Verification items for this drawing (mm, ordinates from the low corner). Round coordinates to 2 decimals unless told otherwise and drop trailing zeros. Loops run counter-clockwise (first coordinate to the right, second up) from the corner with the lowest first, then second, coordinate; pieces in that order, holes last. Notation, with made-up numbers: M 26.5,9.25 L 39.5,9.25 A10 ccw 39.5,26.25 Z; hole C 66.25,37 d4. An arc over 180 degrees is marked long. Answer as CSV lines item,"result".
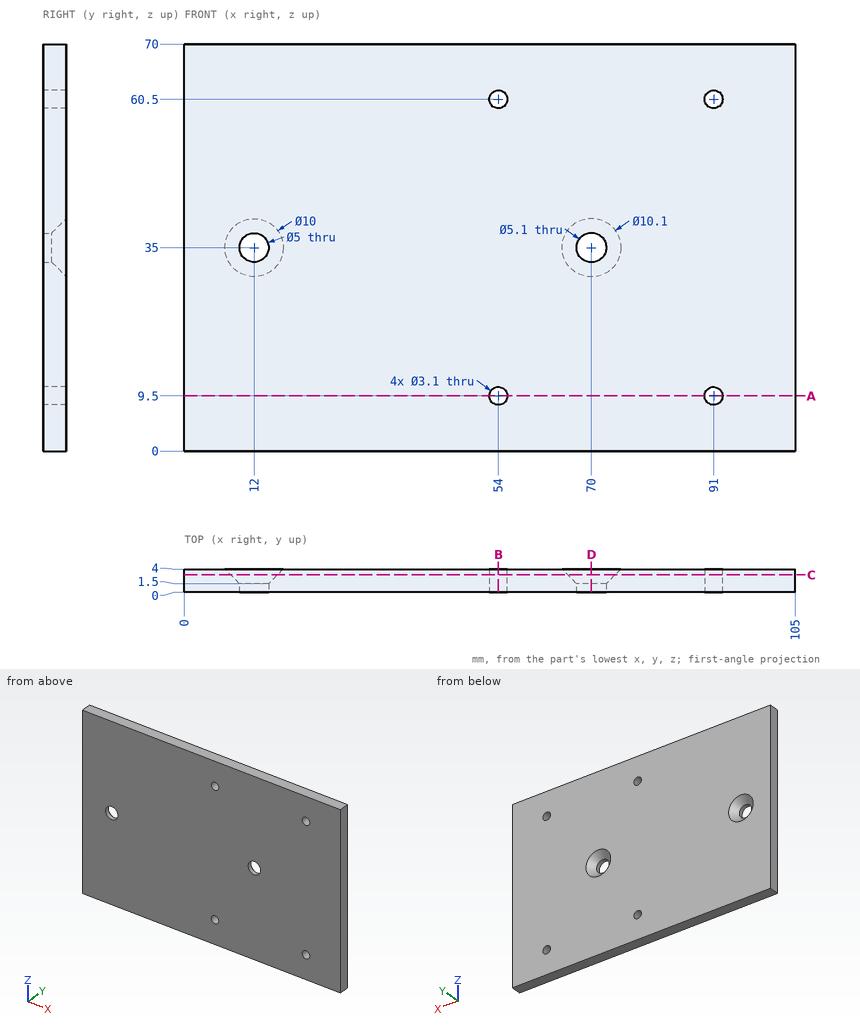
1) Section check D-D (x = 70). Record the cut outline in (y, z).
Here are the results:
outline,"M 0,0 L 4,0 L 4,29.95 L 1.5,32.45 L 0,32.45 Z; M 0,37.55 L 1.5,37.55 L 4,40.05 L 4,70 L 0,70 Z"
2) Go/stop test with flat-tipped pins: pin 1 (2.5 mm diameter, centred on x = 54, z = 60.5, fed in from -Y); pin 2 (8 mm diameter, centred on x = 70, z = 35, fed in from +Y). Record where each tip stops, or that it passes through.
Here are the results:
pin 1,"passes through"
pin 2,"stops at y = 2.95"
3) Section check B-B (x = 54). Record the cut outline in (y, z), plus the area to 3 significant figures.
Here are the results:
outline,"M 0,0 L 4,0 L 4,7.95 L 0,7.95 Z; M 0,11.05 L 4,11.05 L 4,58.95 L 0,58.95 Z; M 0,62.05 L 4,62.05 L 4,70 L 0,70 Z"
area,"255 mm^2"
4) Section check C-C (y = 3). Record the cut outline in (x, z).
Here are the results:
outline,"M 0,0 L 105,0 L 105,70 L 0,70 Z; hole C 12,35 d8; hole C 54,9.5 d3.1; hole C 54,60.5 d3.1; hole C 70,35 d8.1; hole C 91,9.5 d3.1; hole C 91,60.5 d3.1"
5) Section check A-A (z = 9.5). Record the cut outline in (x, y), plus the area to 3 significant figures.
Here are the results:
outline,"M 0,0 L 52.45,0 L 52.45,4 L 0,4 Z; M 55.55,0 L 89.45,0 L 89.45,4 L 55.55,4 Z; M 92.55,0 L 105,0 L 105,4 L 92.55,4 Z"
area,"395 mm^2"
6) Material ranges on probe 1 along X at (y, z) = (0.9, 60.5); probe 2 along Z at (x, y) = (91, 1.4); probe 3 along X at (y, z) = (3.5, 36.5), recorded low to high.
Here are the results:
probe 1,"x = 0 to 52.45, 55.55 to 89.45, 92.55 to 105"
probe 2,"z = 0 to 7.95, 11.05 to 58.95, 62.05 to 70"
probe 3,"x = 0 to 7.76, 16.24 to 65.7, 74.3 to 105"
